Design review of the part shown in the three views and the two pictorial views. Dimensions are in mm from the part's minimum x, y and z. Round coordinates to 2 decimals unless told otherwise and drop trailing zeros. Loops run counter-clockwise (first coordinate to the right, second up) from the corner with the lowest first, then second, coordinate; pieces in that order, holes last. Notation, with made-up numbers: (78, -20) - (104, -20) arc R26 cw to (104, -6) - close; hole circle Ø9 at (89.5, 72.25). An arc over 180 degrees is marked (long way). Return JSON: item names as keys, results as strings. Group by question number.
(1) We need section C-C, the plane y = 7.5. Write out the cut boundary in (x, z).
(2) We need section D-D, the plane y = 2.75. Write out the cut boundary in (x, z).
(3) Wall thickness on L1, parallel to X at y = 3.75, z = 10; L2, parallel to X at y = 12.25, z = 10; L3, parallel to Y at x = 95, z = 15.25: over which ranges is each line inside the solid? List them lowest first. Write a range as [from, to].
(4) We need section B-B, the plane x = 10. Write out the cut boundary in (y, z).
(5) Clearance check with a flat-ended pin moving along its axis: pin 1 (9 mm diameter, centred on x = 90, z = 10, fed in from -Y). State where the tip first meets the part, or that it passes through.
(6) We need section A-A, the plane z = 10. Write out the cut boundary in (x, y).
(7) The part is to be moulded in two halves that separate along X. For the marked faces 1, 2, 3 and 4, say which applies: pulls with the +X half, pulls with the -X half, needs draft (parallel to the pull), parting line crosses it, or undercut.
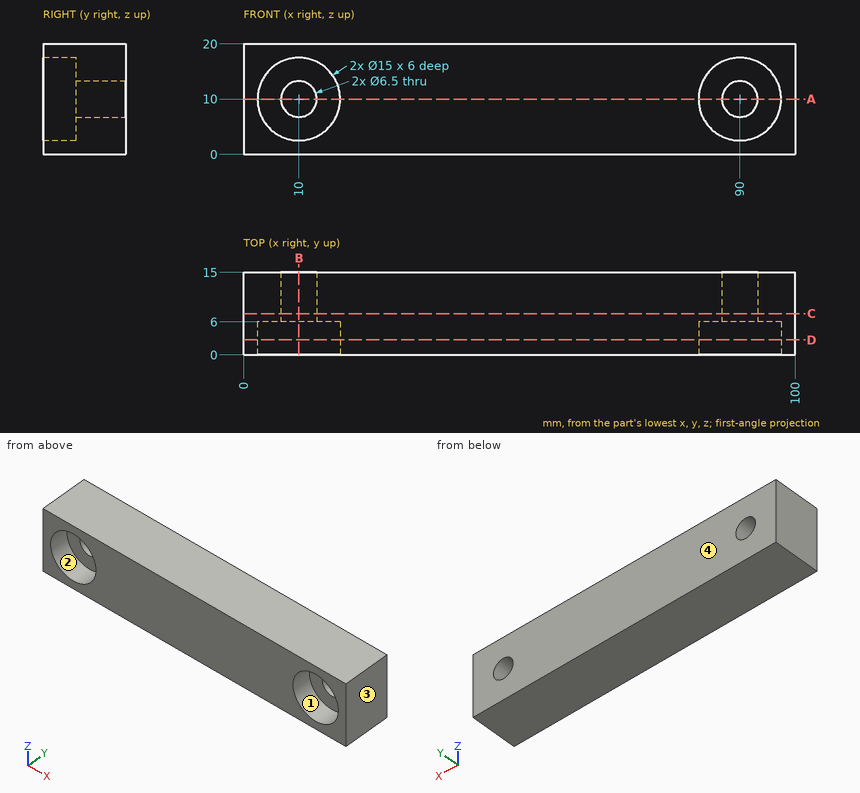
Solutions:
{
 "1": {"outline": "(0, 0) - (100, 0) - (100, 20) - (0, 20) - close; hole circle Ø6.5 at (10, 10); hole circle Ø6.5 at (90, 10)"},
 "2": {"outline": "(0, 0) - (100, 0) - (100, 20) - (0, 20) - close; hole circle Ø15 at (10, 10); hole circle Ø15 at (90, 10)"},
 "3": {"L1": "[0, 2.5], [17.5, 82.5], [97.5, 100]", "L2": "[0, 6.75], [13.25, 86.75], [93.25, 100]", "L3": "[6, 15]"},
 "4": {"outline": "(0, 0) - (15, 0) - (15, 6.75) - (6, 6.75) - (6, 2.5) - (0, 2.5) - close; (0, 17.5) - (6, 17.5) - (6, 13.25) - (15, 13.25) - (15, 20) - (0, 20) - close"},
 "5": {"pin 1": "y = 6"},
 "6": {"outline": "(0, 0) - (2.5, 0) - (2.5, 6) - (6.75, 6) - (6.75, 15) - (0, 15) - close; (13.25, 6) - (17.5, 6) - (17.5, 0) - (82.5, 0) - (82.5, 6) - (86.75, 6) - (86.75, 15) - (13.25, 15) - close; (93.25, 6) - (97.5, 6) - (97.5, 0) - (100, 0) - (100, 15) - (93.25, 15) - close"},
 "7": {"face 1": "undercut", "face 2": "undercut", "face 3": "pulls with the +X half", "face 4": "needs draft"}
}
